The listing builds one solid part. Answer for the finished solid, in the listing's coordinates (mm). Face numbers are marked on the shaded views. A direction names the side the tool comes from. Give positions to 0.01 mm unless a question says otherwise; leave off trailing zeros. Loops run counter-clockwise (first coordinate to the right, second up) from the corner with the lowest first, then second, coordinate; pieces in that order, holes last.
Item 1: Section D-D, the plane y = 82 is taken. Give the vertices of the cut face in (x, z).
Item 2: A tool of negligible diameter and unlimited length cuts with its end or side. For the marked faces 4 and 5, from which of +Z, -Z, +X, -X, +Y, -Y can it reach the whole face along a straight path? Write none if from no direction.
Item 3: Section C-C, the plane y = -91.67 is taken. Give the vertices of the cut face in (x, z), and give its area (3 significant figures).
Item 4: The mould has two halves that part along X. Classify the marked faces 1, 2 and 3: pulls with the +X half, pulls with the -X half, needs draft (parallel to the pull), parting line crosses it, or undercut.
Item 5: Section A-A, the plane z = 33 is taken. Give the vertices of the cut face in (x, y).
Item 6: Each of these flat-tipped pins is pushed along its axis until it touches: pin 1 Ø6 at (x, y) = (16, -32) entering from -Z; pin 2 Ø7 at (x, y) = (59.75, -91.67) entering from +Z. Where does it stop, or does it pass through?
Item 7: Consider line 1 along Y through (x, z) = (-59.75, 75.25); line 2 along X through (y, z) = (-67, -69.5); line 3 along Z through (x, y) = (11, 4). Determine where each line is inside the solid, lowest interval first.
Item 8: Section B-B, the plane x = -59.75 is taken. Give the vertices of the cut face in (y, z).
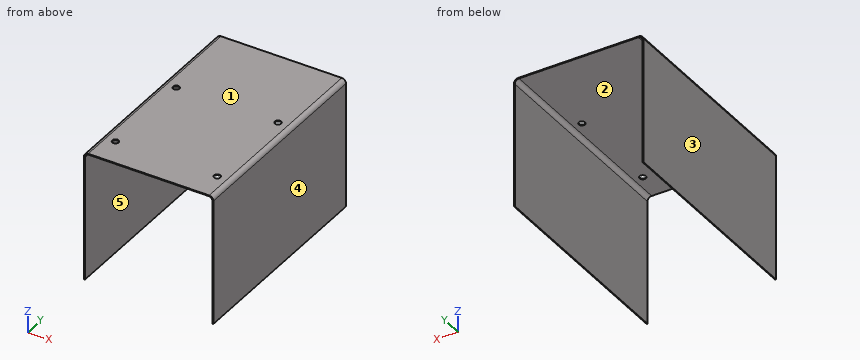
from build123d import *

# Parameters (mm, degrees)
F1_DEPTH = 125
F2_T     = -1
F4_D     = 7.5
F5_R     = 5


with BuildPart() as f1:
    # F0 (on Front) → F1 (new body, symmetric)
    with BuildSketch(Plane.XZ):
        Polygon((76, 76), (0, 76), (-76, 76), (-76, 0), (-76, -76), (0, -76), (76, -76), (76, 0), align=None)
    extrude(amount=F1_DEPTH, both=True)

    # F2
    f2_openings = [f1.faces().sort_by_distance(p)[0] for p in [
        (0, -125, 0),
        (0, 0, -76),
        (0, 125, 0),
    ]]
    offset(amount=F2_T, openings=f2_openings)

    # F4 (through all)
    with Locations(Plane.XY.offset(76)):
        with Locations((-59.75, 22.88), (59.75, 22.88), (59.75, -91.67), (-59.75, -91.67)):
            Hole(F4_D / 2)

    # F5
    f5_edges = [f1.edges().sort_by_distance(p)[0] for p in [
        (-75, 0, 75),
        (75, 0, 75),
        (76, 0, 76),
        (-76, 0, 76),
    ]]
    fillet(f5_edges, radius=F5_R)


solid = f1.part
Worked answers:
1. outline: (-76, -76) - (-75, -76) - (-75, 70) arc R5 cw to (-70, 75) - (70, 75) arc R5 cw to (75, 70) - (75, -76) - (76, -76) - (76, 71) arc R5 ccw to (71, 76) - (-71, 76) arc R5 ccw to (-76, 71) - close
2. face 4: +Z, -Z, +X, +Y, -Y
2. face 5: -Z, +Y, -Y
3. outline: (-76, -76) - (-75, -76) - (-75, 70) arc R5 cw to (-70, 75) - (-63.5, 75) - (-63.5, 76) - (-71, 76) arc R5 ccw to (-76, 71) - close; (-56, 75) - (56, 75) - (56, 76) - (-56, 76) - close; (63.5, 75) - (70, 75) arc R5 cw to (75, 70) - (75, -76) - (76, -76) - (76, 71) arc R5 ccw to (71, 76) - (63.5, 76) - close
3. area: 439 mm2
4. face 1: needs draft
4. face 2: undercut
4. face 3: pulls with the -X half
5. outline: (-76, -125) - (-75, -125) - (-75, 125) - (-76, 125) - close; (75, -125) - (76, -125) - (76, 125) - (75, 125) - close
6. pin 1: stops at z = 75
6. pin 2: passes through
7. line 1: y = -125 to -95.42, -87.92 to 19.13, 26.63 to 125
7. line 2: x = -76 to -75, 75 to 76
7. line 3: z = 75 to 76
8. outline: (-125, 75) - (-95.42, 75) - (-95.42, 76) - (-125, 76) - close; (-87.92, 75) - (19.13, 75) - (19.13, 76) - (-87.92, 76) - close; (26.63, 75) - (125, 75) - (125, 76) - (26.63, 76) - close
